Print and shaded views of the part. All mm, measured from the part's lowest x, y and z. A direction names the side the tool comes from. Give positions to 0.01 mm unless a question says otherwise; leave off trailing zeros. Order: outer loops, then holes, each group sorted by start corner. A loop starts at its lowest first (then second) coordinate and runs counter-clockwise, first axis right, second up. Notation, with made-up numbers: (52, 65.25) -> (111, 65.25) arc R29 cw to (111, 97.25) -> close; hole circle Ø5 at (14.5, 34). An arc over 180 degrees is marked (long way). One line per question, with ' | ' between items. Start each with the question number.
(1) Pin check, flat tips, straight feed: pin 1 Ø3 at (x, z) = (9, 4.5) entering from -Y; pin 2 Ø2 at (x, y) = (20.5, 8) entering from +Z. Stop position of each tip, or through.
(2) Cut at B-B (x = 33). Give the cut face in (y, z).
(3) Drill centre lines: L1, parallel to X at y = 10.5, z = 7.75; L2, parallel to Y at x = 24, z = 8.25; L3, parallel to Y at x = 26, z = 3.25. Where is each one in solid material? Low to high. Write a range as from..to.
(4) Cut at C-C (y = 5.75). Give the cut face in (x, z).
(5) Cut at A-A (z = 5). Give the cut face in (x, y), then the cut area to 3 significant figures.
(6) Which spindle directions (+Z, -Z, +X, -X, +Y, -Y) get a long thin tool onto all of the face, cutting with end or side? Do the marked faces 1, 2 and 3. Say none if no direction does.
(7) Cut at D-D (x = 27.5). Give the cut face in (y, z).
(8) Pull direction X, two halves, no side cores. Call the marked faces 4, 5, 6 and 7: +X half, -X half, draft (parallel to the pull), parting line (faces both ways), or undercut.
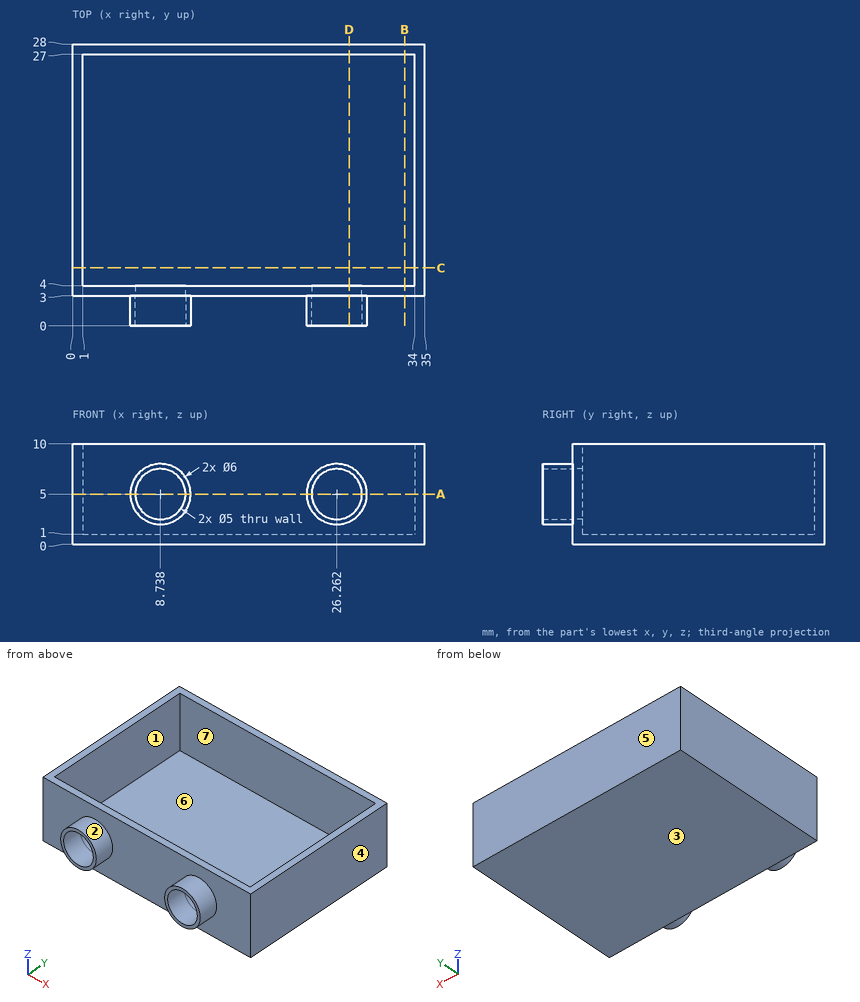
Result set:
1) pin 1: stops at y = 27 | pin 2: stops at z = 1
2) outline: (3, 0) -> (28, 0) -> (28, 10) -> (27, 10) -> (27, 1) -> (4, 1) -> (4, 10) -> (3, 10) -> close
3) L1: x = 0..1, 34..35 | L2: y = 3..4, 27..28 | L3: y = 27..28
4) outline: (0, 0) -> (35, 0) -> (35, 10) -> (34, 10) -> (34, 1) -> (1, 1) -> (1, 10) -> (0, 10) -> close
5) outline: (0, 3) -> (5.74, 3) -> (5.74, 0) -> (6.24, 0) -> (6.24, 4) -> (1, 4) -> (1, 27) -> (34, 27) -> (34, 4) -> (28.76, 4) -> (28.76, 0) -> (29.26, 0) -> (29.26, 3) -> (35, 3) -> (35, 28) -> (0, 28) -> close; (11.24, 0) -> (11.74, 0) -> (11.74, 3) -> (23.26, 3) -> (23.26, 0) -> (23.76, 0) -> (23.76, 4) -> (11.24, 4) -> close | area: 112 mm2
6) face 1: +Z | face 2: -Y | face 3: -Z, +X, -X, +Y, -Y
7) outline: (0, 2.27) -> (3, 2.27) -> (3, 0) -> (28, 0) -> (28, 10) -> (27, 10) -> (27, 1) -> (4, 1) -> (4, 2.83) -> (0, 2.83) -> close; (0, 7.17) -> (4, 7.17) -> (4, 10) -> (3, 10) -> (3, 7.73) -> (0, 7.73) -> close
8) face 4: +X half | face 5: draft | face 6: undercut | face 7: undercut
